from build123d import *

# Parameters (mm, degrees)
SKETCH2_OUTSIDE_W = 16.808
SKETCH2_OUTSIDE_H = 16.808
EXTRUDE2_DEPTH    = 15.748315158


with BuildPart() as part:
    # Sketch1 → Revolve1 (revolve)
    with BuildSketch(Plane(origin=(0, 0, 0), x_dir=(0, 0, -1), z_dir=(1, 0, 0)), mode=Mode.PRIVATE) as revolve1_sk:
        Polygon((0, 0), (0, 3.5), (-0.514462449, 5.42), (-7.35, 5.42), (-7.35, 4.66), (-10.05, 4.66), (-10.05, 5.42), (-12.6, 5.42), (-12.6, 4.1), (-11.35, 4.1), (-11.35, 3.45), (-6.5, 3.45), (-6.5, 1.5), (-4.801290929, 1.5), (-3.9, 0), align=None)
    revolve(revolve1_sk.sketch.rotate(Axis((0, 0, 0), (0, 0, 1)), 90), axis=Axis((0, 0, 0), (0, 0, 1)))

    # Sketch2 outside → Extrude2 (cut, through all)
    with BuildSketch(Plane(origin=(0, 0, 0), x_dir=(-1, 0, 0), z_dir=(0, 0, -1))):
        Rectangle(SKETCH2_OUTSIDE_W, SKETCH2_OUTSIDE_H)
        Polygon((4.825, 2.785715049), (0, 5.571430098), (-4.825, 2.785715049), (-4.825, -2.785715049), (0, -5.571430098), (4.825, -2.785715049), align=None, mode=Mode.SUBTRACT)
    extrude(amount=-EXTRUDE2_DEPTH, mode=Mode.SUBTRACT)


solid = part.part
Input: part model. Units: mm. Frame: model coordinates. A direction names the side the tool comes from. Give positions to 0.01 mm unless a question says otherwise; leave off trailing zeros. Order: outer loops, then holes, each group sorted by start corner. A loop starts at its lowest first (then second) coordinate and runs counter-clockwise, first axis right, second up. Notation, with made-up numbers: (-15.5, 66.25) - (20.5, 66.25) arc R14 cw to (20.5, 71.25) - close; hole circle Ø2 at (-37.75, 64). An arc over 180 degrees is marked (long way). Answer as a JSON object with one key per item and string values. Group by question number.
Q1. Cut plane B-B, the plane z = 4.25. Output: boundary loops of the cut face in (x, y) (1 decimal).
Q2. Set-up query: faces 1 (the face through (4, 2, 12.6)), 2 (the face through (-1.43, -0.45, 5.64)). Return all of +Z, -Z, +X, -X, +Y, -Y with unobstructed straight access to the full face (end or side cutting, diameter ignored); none if empty.
Q3. Line query: probe 1 along Z at (x, y) = (-1.5, 1.5); probe 2 along X at (y, z) = (2, 12) (3 decimals); probe 3 along X at (y, z) = (-0.5, 12) (3 decimals). Output: solid intervals per line, ascending.
Q4. Mould query, pull axis Z, two halves, no side actions, for faces 3 (the face through (0, 0, 0)), 4 (the face through (-2.383, -4.196, 11.307)), 5 (the face through (-4.445, -1.4, 8.719)). Classes: pulls with the +Z half, pulls with the -Z half, needs draft (parallel to the pull), parting line crosses it, or undercut.
Q5. First-contact query: pin 1 Ø5 at (x, y) = (0, 0) entering from +Z; pin 2 Ø3 at (x, z) = (3, 11) entering from -Y. Flat tips, straight axial feed; report the tip coordinate or a pass-through.
Q6. Cut plane A-A, the plane z = 1. Output: boundary loops of the cut face in (x, y) (3 decimals).
Results:
{
 "1": {"outline": "(-4.8, -2.5) arc R5.4 ccw to (-4.6, -2.9) - (-0.3, -5.4) arc R5.4 ccw to (0.3, -5.4) - (4.6, -2.9) arc R5.4 ccw to (4.8, -2.5) - (4.8, 2.5) arc R5.4 ccw to (4.6, 2.9) - (0.3, 5.4) arc R5.4 ccw to (-0.3, 5.4) - (-4.6, 2.9) arc R5.4 ccw to (-4.8, 2.5) - close; hole circle Ø1.2 at (0, 0)"},
 "2": {"face 1": "+Z, +X, -X, +Y, -Y", "face 2": "+Z"},
 "3": {"probe 1": "0 to 6.5", "probe 2": "-4.825 to -3.579, 3.579 to 4.825", "probe 3": "-4.825 to -4.069, 4.069 to 4.825"},
 "4": {"face 3": "pulls with the -Z half", "face 4": "needs draft", "face 5": "undercut"},
 "5": {"pin 1": "z = 6.5", "pin 2": "y = -4.71"},
 "6": {"outline": "(-4.825, -2.469) arc R5.42 ccw to (-4.551, -2.944) - (-0.274, -5.413) arc R5.42 ccw to (0.274, -5.413) - (4.551, -2.944) arc R5.42 ccw to (4.825, -2.469) - (4.825, 2.469) arc R5.42 ccw to (4.551, 2.944) - (0.274, 5.413) arc R5.42 ccw to (-0.274, 5.413) - (-4.551, 2.944) arc R5.42 ccw to (-4.825, 2.469) - close"}
}
